Source: CAD feature listing. Evaluate the final solid. Frame: model axes, mm. A direction names the side the tool comes from. Coordinates: 2 decimals unless noted, no trailing zeros. Write each loop counter-clockwise with the first axis right and the second up, starting at its lowest first coordinate (ties: lowest second). Pieces come first, ordered by that corner, then holes. Notation, with made-up numbers: (46.25, 45) - (94.25, 45) arc R14 ccw to (94.25, 65) - close; hole circle Ø10 at (46, -9). An arc over 180 degrees is marked (long way). One line per item, written item: value.
from build123d import *

# Parameters (mm, degrees)
BOSS_EXTRUDE1_DEPTH = 20
FILLET2_R           = 2
FILLET3_R           = 9
FILLET1_R           = 1
HOLE1_D             = 5.3


with BuildPart() as part:
    # Sketch2 → Boss-Extrude1 (new body, symmetric)
    with BuildSketch(Plane.XY):
        Polygon((0, 0), (-35, 0), (-35, 7), (-8.342275148, 7), (-16.965248576, 55.903312431), (-10.071594305, 57.118849675), align=None)
    extrude(amount=BOSS_EXTRUDE1_DEPTH, both=True)

    # Fillet2
    fillet2_edges = [part.edges().sort_by_distance(p)[0] for p in [
        (-8.342275148, 7, 0),
    ]]
    fillet(fillet2_edges, radius=FILLET2_R)

    # Fillet3
    fillet3_edges = [part.edges().sort_by_distance(p)[0] for p in [
        (0, 0, 0),
    ]]
    fillet(fillet3_edges, radius=FILLET3_R)

    # Fillet1
    fillet1_edges = [part.edges().sort_by_distance(p)[0] for p in [
        (-35, 0, 0),
        (-35, 7, 0),
        (-16.965248576, 55.903312431, 0),
        (-10.071594305, 57.118849675, 0),
        (-12.860707702, 32.625304393, 20),
        (-22.862891167, 7, -20),
        (-22.862891167, 7, 20),
        (-35, 3.5, 20),
        (-9.193693447, 7.714424781, -20),
        (-9.193693447, 7.714424781, 20),
        (-22.862891167, 0, 20),
        (-5.96705343, 33.840841637, -20),
        (-5.96705343, 33.840841637, 20),
        (-3.831382345, 3.214911513, -20),
        (-3.831382345, 3.214911513, 20),
        (-22.862891167, 0, -20),
        (-35, 3.5, -20),
        (-12.860707702, 32.625304393, -20),
        (-13.51842144, 56.511081053, -20),
        (-13.51842144, 56.511081053, 20),
    ]]
    fillet(fillet1_edges, radius=FILLET1_R)

    # Hole1 (through all)
    with Locations(Plane(origin=(0, 0, 0), x_dir=(0, 0, -1), z_dir=(0.984807753, 0.173648178, 0))):
        with Locations((0, 50.31616731), (0, 15.31616731)):
            Hole(HOLE1_D / 2)


solid = part.part
1) Draft query along Z for faces 1 (the cylindrical face through (-5.75, 12.15, 1.22)), 2 (the cylindrical face through (-6.12, 32.977, 19.715)), 3 (the cylindrical face through (-9.18, 7.73, -0.27)), 4 (the cylindrical face through (-13.434, 56.236, -19.699)). Return one class per face: released by +Z, released by -Z, zero draft, split by the parting line, or undercut.
Values found:
face 1: undercut
face 2: released by +Z
face 3: zero draft
face 4: released by -Z
2) Contact query for flat-ended pins moving along their axis: P1, Ø8, axis at x = -7, z = 1.5, coming from the -Y side; P2, Ø3, axis at y = 42.5, z = 9.5, coming from the -X side; P3, Ø4, axis at x = -26.5, z = 15.5, coming from the +Y side; P4, Ø12, axis at y = 18.5, z = -10, coming from the +X side. Output: stop coordinate, or through.
Values found:
P1: y = 0
P2: x = -14.87
P3: y = 7
P4: x = -2.2
3) Reachability of faces 5 (the cylindrical face through (-13.432, 56.221, 19.715)), 6 (the cylindrical face through (-12.55, 32.5, -19.7)), 7 (the flat face through (-23, 7, 0)), 8 (the flat face through (-5.936, 33.667, 0.266)), 9 (the cylindrical face through (-12.534, 32.504, 19.715)) from +Z, -Z, +X, -X, +Y, -Y: full face, straight path, thin tool, end or side. Return the list, or none.
Values found:
face 5: +Z, -X, +Y
face 6: -Z, -X
face 7: +Z, -Z, -X
face 8: +Z, -Z, +X, +Y
face 9: +Z, -X
4) Material intervals for line 1 (Y direction, x = -16, z = -1); line 2 (Y direction, x = -28, z = -14); line 3 (X direction, y = 53, z = -16.5), sorted ascending.
Values found:
line 1: 0 to 7, 50.76 to 56.07
line 2: 0 to 7
line 3: -16.45 to -9.35
5) Section query B-B on z = 10.5. Output: boundary loops of the cut face in (x, y), then the cut area to 3 significant figures.
Values found:
outline: (-35, 1) arc R1 ccw to (-34, 0) - (-10.73, 0) arc R9 ccw to (-1.86, 10.56) - (-9.9, 56.13) arc R1 ccw to (-11.06, 56.95) - (-15.98, 56.08) arc R1 ccw to (-16.79, 54.92) - (-8.76, 9.35) arc R2 cw to (-10.73, 7) - (-34, 7) arc R1 ccw to (-35, 6) - close
area: 567 mm2
6) Section query A-A on x = -23. Output: boundary loops of the cut face in (y, z), then the cut area to 3 significant figures.
Values found:
outline: (0, -19) arc R1 ccw to (1, -20) - (6, -20) arc R1 ccw to (7, -19) - (7, 19) arc R1 ccw to (6, 20) - (1, 20) arc R1 ccw to (0, 19) - close
area: 279 mm2
